from build123d import *

# Parameters (mm, degrees)
PAD_DEPTH            = 13.4
POCKET001_DEPTH      = 8.4
POCKET001_DEPTH_BACK = 100
SKETCH003_R          = 2.6
POCKET002_DEPTH      = 24.4921624319
SKETCH004_R          = 5.25
POCKET_DEPTH         = 25
SKETCH007_W          = 3
SKETCH007_H          = 2
PAD001_DEPTH         = 1.6
PAD001_DEPTH_BACK    = 4
POCKET005_DEPTH      = 8.25
PAD002_DEPTH         = 13.4
POCKET006_DEPTH      = 5
SKETCH010_R          = 4.25
POCKET007_DEPTH      = 5
CHAMFER_SIZE         = 4
CHAMFER001_SIZE      = 2
FILLET_R             = 6
SKETCH011_R          = 1.6
POCKET008_DEPTH      = 16
POCKET009_DEPTH      = 6
SKETCH013_W          = 8
SKETCH013_H          = 7
POCKET010_DEPTH      = 2
FILLET001_R          = 1
PAD003_DEPTH         = 14
PAD004_DEPTH         = 8.25
POCKET011_DEPTH      = 15


with BuildPart() as part:
    # Sketch → Pad (new body)
    with BuildSketch(Plane.XY):
        Polygon((0, 0), (0, 20), (5, 20), (5, -5), (-24.3031833154, -24.4911624319), (-27.5797914926, -22.1968566865), (-18.6893567291, -9.5), (-20, -8.5822777018), (-20, 0), align=None)
    extrude(amount=PAD_DEPTH)

    # Sketch002 → Pocket001 (cut, two sides)
    with BuildSketch(Plane.XY.offset(13.4)) as pocket001_sk:
        Polygon((14.314081, -22.145182), (14.314081, 26.828188), (0, 26.828188), (0, 0), (0, -22.145182), align=None)
    extrude(amount=-POCKET001_DEPTH, mode=Mode.SUBTRACT)
    extrude(pocket001_sk.sketch, amount=POCKET001_DEPTH_BACK, mode=Mode.SUBTRACT)

    # Sketch003 → Pocket002 (cut, through all)
    with BuildSketch(Plane.XZ):
        with Locations((-10, 7.5)):
            Circle(SKETCH003_R)
    extrude(amount=POCKET002_DEPTH, mode=Mode.SUBTRACT)

    # Sketch004 (on DatumPlane) → Pocket (cut)
    with BuildSketch(Plane(origin=(0, -30, 0), x_dir=(-1, 0, 0), z_dir=(0, 1, 0))):
        with Locations((10, 7.5)):
            Circle(SKETCH004_R)
    extrude(amount=POCKET_DEPTH, mode=Mode.SUBTRACT)

    # Sketch007 (on DatumPlane) → Pad001 (join, two sides)
    with BuildSketch(Plane(origin=(-8.0772066494, 5.6557209836, 0), x_dir=(-0.5735764364, -0.8191520443, 0), z_dir=(-0.8191520443, 0.5735764364, 0))) as pad001_sk:
        with Locations((35.5, 1)):
            Rectangle(SKETCH007_W, SKETCH007_H)
    extrude(amount=PAD001_DEPTH)
    extrude(pad001_sk.sketch, amount=-PAD001_DEPTH_BACK)

    # Sketch008 (on DatumPlane) → Pocket005 (cut)
    with BuildSketch(Plane.XY.offset(13.4)):
        Polygon((-15.88, -5), (-14.38, 0), (-20, 0), (-20, -8.59), (-15.88, -11.4748550574), (-15.88, -25), (-3.690549763, -25), (0, -25), (0, -10), (0, -5), align=None)
    extrude(amount=-POCKET005_DEPTH, mode=Mode.SUBTRACT)

    # Sketch009 → Pad002 (join)
    with BuildSketch(Plane.XY):
        Polygon((-14.375, 0), (-13, 1.85), (-7, 1.85), (-5.625, 0), align=None)
    extrude(amount=PAD002_DEPTH)

    # Sketch003 → Pocket006 (cut)
    with BuildSketch(Plane.XZ):
        with Locations((-10, 7.5)):
            Circle(SKETCH003_R)
    extrude(amount=-POCKET006_DEPTH, mode=Mode.SUBTRACT)

    # Sketch010 → Pocket007 (cut)
    with BuildSketch(Plane.XZ):
        with Locations((-10, 7.5)):
            Circle(SKETCH010_R)
    extrude(amount=-POCKET007_DEPTH, mode=Mode.SUBTRACT)

    # Chamfer
    chamfer_edges = [part.edges().sort_by_distance(p)[0] for p in [
        (5, 20, 2.5),
    ]]
    chamfer(chamfer_edges, length=CHAMFER_SIZE)

    # Chamfer001
    chamfer001_edges = [part.edges().sort_by_distance(p)[0] for p in [
        (0.5, 20, 5),
        (0.5, 20, 0),
    ]]
    chamfer(chamfer001_edges, length=CHAMFER001_SIZE)

    # Fillet
    fillet_edges = [part.edges().sort_by_distance(p)[0] for p in [
        (5, 16, 2.5),
    ]]
    fillet(fillet_edges, radius=FILLET_R)

    # Sketch011 (on DatumPlane) → Pocket008 (cut)
    with BuildSketch(Plane(origin=(-0.7048382508, 0.4935330564, 0), x_dir=(-0.5735764364, -0.8191520443, 0), z_dir=(-0.8191520443, 0.5735764364, 0))):
        with Locations((30.3, 9.5)):
            Circle(SKETCH011_R)
    extrude(amount=POCKET008_DEPTH, mode=Mode.SUBTRACT)

    # Sketch012 (on DatumPlane) → Pocket009 (cut)
    with BuildSketch(Plane(origin=(-0.7048382508, 0.4935330564, 0), x_dir=(-0.5735764364, -0.8191520443, 0), z_dir=(-0.8191520443, 0.5735764364, 0))):
        Polygon((33.05, 7.9122867597), (33.05, 11.0877132403), (30.3, 12.6754264805), (27.55, 11.0877132403), (27.55, 7.9122867597), (30.3, 6.3245735195), align=None)
    extrude(amount=POCKET009_DEPTH, mode=Mode.SUBTRACT)

    # Sketch013 (on DatumPlane) → Pocket010 (cut)
    with BuildSketch(Plane(origin=(-8.0772066494, 5.6557209836, 0), x_dir=(-0.5735764364, -0.8191520443, 0), z_dir=(-0.8191520443, 0.5735764364, 0))):
        with Locations((23.5, 8.5)):
            Rectangle(SKETCH013_W, SKETCH013_H)
    extrude(amount=-POCKET010_DEPTH, mode=Mode.SUBTRACT)

    # Fillet001
    fillet001_edges = [part.edges().sort_by_distance(p)[0] for p in [
        (4.543277, 15.810819, 5),
        (4.543277, 15.810819, 0),
    ]]
    fillet(fillet001_edges, radius=FILLET001_R)

    # Fillet001 Face52 → Pad003 (add)
    with BuildSketch(Plane(origin=(-5.7758983743, -5, 10.0600347273), x_dir=(-1, 0, 0), z_dir=(0, -1, 0))):
        with BuildLine():
            Line((-5.7758983743, -3.3399652727), (10.1041016257, -3.3399652727))
            Line((10.1041016257, -3.3399652727), (10.1041016257, 4.9100347273))
            Line((10.1041016257, 4.9100347273), (8.9187794634, 4.9100347273))
            ThreePointArc((8.9187794634, 4.9100347273), (9.3333852666, 3.7673957652), (9.4741016257, 2.5600347273))
            ThreePointArc((9.4741016257, 2.5600347273), (3.0167405877, -2.5492489137), (-0.4705762121, 4.9100347273))
            Line((-0.4705762121, 4.9100347273), (-5.7758983743, 4.9100347273))
            Line((-5.7758983743, 4.9100347273), (-5.7758983743, -3.3399652727))
        make_face()
    extrude(amount=PAD003_DEPTH)

    # Sketch014 (on Face41 of Pad003) → Pad004 (join)
    with BuildSketch(Plane.XY.offset(5.15)):
        Polygon((-15.88, -5), (-20, -8.5822777018), (-15.88, -11.4748550574), align=None)
    extrude(amount=PAD004_DEPTH)

    # Sketch015 → Pocket011 (cut)
    with BuildSketch(Plane.XY):
        Polygon((-15.88, -18.8884389179), (-17.149737, -23.146951), (5.036606, -23.146951), (0, -8.325775603), align=None)
    extrude(amount=POCKET011_DEPTH, mode=Mode.SUBTRACT)


solid = part.part
Geometry check sheet. Reference: the model listing, model coordinates, mm. A direction names the side the tool comes from. Round coordinates to 2 decimals unless told otherwise and drop trailing zeros. Order: outer loops, then holes, each group sorted by start corner. A loop starts at its lowest first (then second) coordinate and runs counter-clockwise, first axis right, second up. Notation, with made-up numbers: M -29.75,78 L -9.75,78 A21 cw -9.75,106 Z; hole C 7.5,-28 d1. An arc over 180 degrees is marked long. Answer in a Markdown table with one row per item. Add a question column.
Item 1: Set-up check for faces 1 (the face through (-10.1, 0, 4.7)), 2 (the face through (2, 5, 5)), 3 (the face through (-23.005, -22.583, 11.87)), 4 (the face through (-17, 0, 2)): record each of +Z, -Z, +X, -X, +Y, -Y from which the full face is reachable in a straight line by a thin tool's end or side.
Item 2: Draft check along Z on faces 5 (the face through (-13.132, 0.649, 10.372)), 6 (the face through (4.715, 3.791, 4.699)), 7 (the face through (4.699, 3.791, 0.285)). Enter one of: released by +Z, released by -Z, zero draft, split by the parting line, or undercut.
Item 3: Sectioned sample at B-B, the plane x = -1.5. Enter the section's corners in (y, z).
Item 4: Depth check by flat-ended pin: pin 1 Ø8 at (x, y) = (-6, -16) entering from +Z; pin 2 Ø4 at (y, z) = (-5, 2) entering from -X; pin 3 Ø5 at (x, z) = (-5, 2) entering from -Y; pin 4 Ø5.5 at (y, z) = (11.5, 1.5) entering from -X. Enter the tip coordinate at first touch or a pass-through.
Item 5: Material ranges on L1, parallel to Z at x = -10, y = 1.1; L2, parallel to Z at x = -10, y = -13; L3, parallel to Y at x = -24.5, z = 10.5, recorded low to high. Write a range as [from, to].
Item 6: Sectioned sample at A-A, the plane x = -10. Enter the section's corners in (y, z).
Filled in:
| question | item | result |
|---|---|---|
| 1 | face 1 | +Y |
| 1 | face 2 | +Z, +X, +Y, -Y |
| 1 | face 3 | none |
| 1 | face 4 | +Z, -Z, -X, +Y |
| 2 | face 5 | undercut |
| 2 | face 6 | released by +Z |
| 2 | face 7 | released by -Z |
| 3 | outline | M -9.32,0 L 0,0 L 0,13.4 L -9.32,13.4 Z |
| 4 | pin 1 | stops at z = 13.4 |
| 4 | pin 2 | stops at x = -20 |
| 4 | pin 3 | stops at y = -13.31 |
| 4 | pin 4 | stops at x = 0 |
| 5 | L1 | z = [0, 3.25], [11.75, 13.4] |
| 5 | L2 | z = [0, 2.25], [12.75, 13.4] |
| 5 | L3 | y = [-24.35, -23.19], [-23.03, -21.36], [-18.31, -17.8] |
| 6 | outline | M -14.98,0 L 1.85,0 L 1.85,3.25 L 0,3.25 L 0,4.9 L -5,4.9 L -5,2.25 L -14.98,2.25 Z; M -14.98,12.75 L -5,12.75 L -5,10.1 L 0,10.1 L 0,11.75 L 1.85,11.75 L 1.85,13.4 L -14.98,13.4 Z |
